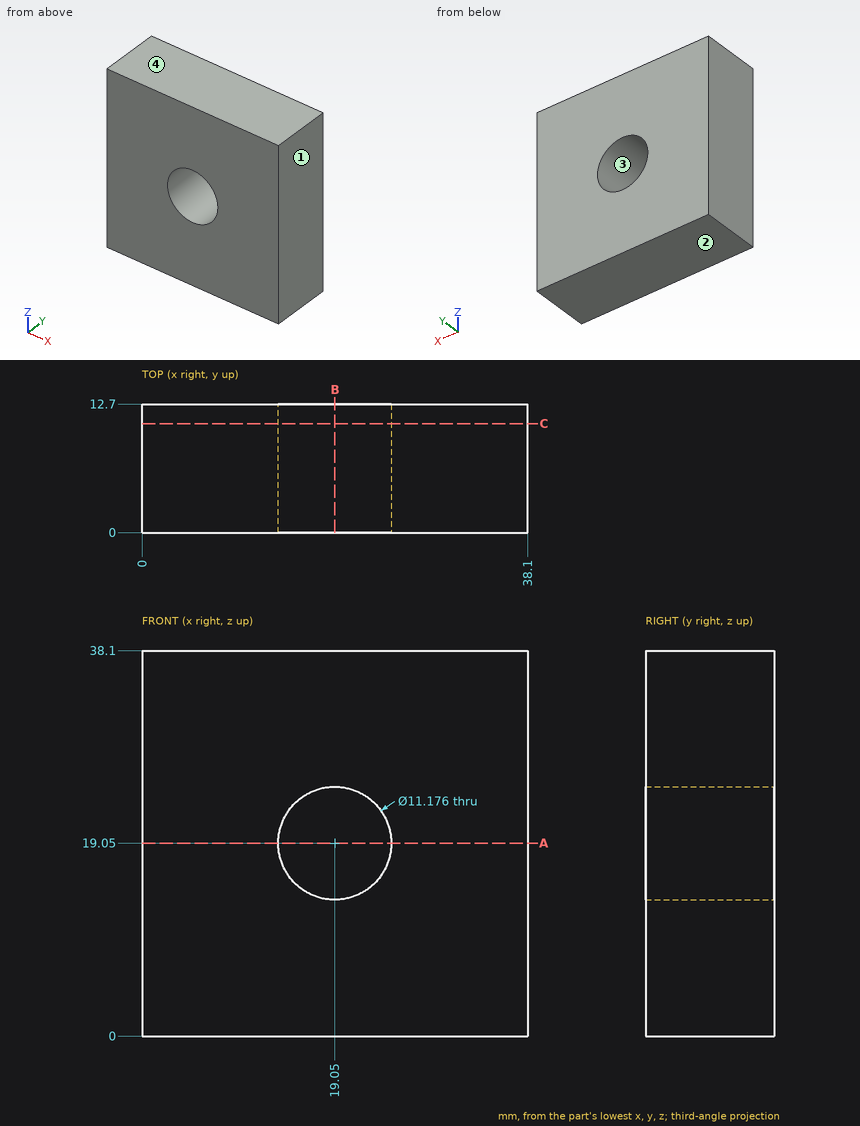
Geometry: see drawing. Coordinates: mm, zero at the bounding-box minimum. Round coordinates to 2 decimals unless told otherwise and drop trailing zeros. Write each loop counter-clockwise with the first axis right and the second up, starting at its lowest first coordinate (ties: lowest second). Pieces come first, ordered by that corner, then holes. Notation, with made-up numbers: M 9,-20 L 32,-20 A21 cw 32,17 Z; hole C 72.5,14 d4. An arc over 180 degrees is marked long. Answer in a Markdown table with one row per item. Add a question column.
(1) Cut plane B-B, the plane x = 19.05. Return the cut outline in (y, z), then the cut area to 3 significant figures.
(2) Draft query along Z for the marked faces 1, 2, 3 and 4. Return one class per face: pulls with the +Z half, pulls with the -Z half, needs draft (parallel to the pull), parting line crosses it, or undercut.
(3) Cut plane A-A, the plane z = 19.05. Return the cut outline in (x, y), then the cut area to 3 significant figures.
(4) Cut plane C-C, the plane y = 10.75. Return the cut outline in (x, z), then the cut area to 3 significant figures.
(5) Ray query, L1, parallel to X at y = 9, z = 19.05; L2, parallel to X at y = 6.5, z = 15. Return the intervals inside material, ascending.
Established:
| question | item | result |
|---|---|---|
| 1 | outline | M 0,0 L 12.7,0 L 12.7,13.46 L 0,13.46 Z; M 0,24.64 L 12.7,24.64 L 12.7,38.1 L 0,38.1 Z |
| 1 | area | 342 mm² |
| 2 | face 1 | needs draft |
| 2 | face 2 | pulls with the -Z half |
| 2 | face 3 | undercut |
| 2 | face 4 | pulls with the +Z half |
| 3 | outline | M 0,0 L 13.46,0 L 13.46,12.7 L 0,12.7 Z; M 24.64,0 L 38.1,0 L 38.1,12.7 L 24.64,12.7 Z |
| 3 | area | 342 mm² |
| 4 | outline | M 0,0 L 38.1,0 L 38.1,38.1 L 0,38.1 Z; hole C 19.05,19.05 d11.18 |
| 4 | area | 1,350 mm² |
| 5 | L1 | 0 to 13.46, 24.64 to 38.1 |
| 5 | L2 | 0 to 15.2, 22.9 to 38.1 |
